Can you work these out from the model? Positions are in its coordinate system, mm. Round coordinates to 2 decimals unless told otherwise and drop trailing zeros. Loops run counter-clockwise (first coordinate to the right, second up) from the corner with the lowest first, then second, coordinate; pieces in that order, holes last. Notation, with made-up numbers: (62, 40.5) -> (98, 40.5) arc R9 cw to (98, 57.5) -> close; hole circle Ø4 at (27.5, 11). An arc over 180 degrees is marked (long way). Answer as a JSON object with one key per item and string values.
```python
from build123d import *

# Parameters (mm, degrees)
SKETCH_1_W          = 130
SKETCH_1_H          = 130
EXTRUDE_1_DEPTH     = 3
SKETCH_5_R          = 2
CUT_EXTRUDE_4_DEPTH = 3
SKETCH_6_R          = 1.5
SKETCH_6_R_2        = 1.464964174
CUT_EXTRUDE_5_DEPTH = 10


with BuildPart() as part:
    # 草图1 → 凸台-拉伸1 (new body)
    with BuildSketch(Plane.XY):
        Rectangle(SKETCH_1_W, SKETCH_1_H)
    extrude(amount=EXTRUDE_1_DEPTH)

    # 草图5 → 切除-拉伸4 (cut)
    with BuildSketch(Plane.XY.offset(3)):
        with Locations((25, -25)):
            Circle(SKETCH_5_R)
        with Locations((-25, 25)):
            Circle(SKETCH_5_R)
    extrude(amount=-CUT_EXTRUDE_4_DEPTH, mode=Mode.SUBTRACT)

    # 草图6 → 切除-拉伸5 (cut)
    with BuildSketch(Plane.XY.offset(3)):
        with Locations((-54.393398282, 54.393398282)):
            Circle(SKETCH_6_R)
        with Locations((-43.786796564, 43.786796564)):
            Circle(SKETCH_6_R)
        with Locations((-10.232887384, 47)):
            Circle(SKETCH_6_R)
        with Locations((9.767112616, 47)):
            Circle(SKETCH_6_R)
        with Locations((43.786796564, 43.786796564)):
            Circle(SKETCH_6_R)
        with Locations((54.393398282, 54.393398282)):
            Circle(SKETCH_6_R)
        with Locations((-47, 10)):
            Circle(SKETCH_6_R)
        with Locations((-47, -10)):
            Circle(SKETCH_6_R)
        with Locations((47, -10)):
            Circle(SKETCH_6_R)
        with Locations((47, 10)):
            Circle(SKETCH_6_R)
        with Locations((-54.393398282, -54.393398282)):
            Circle(SKETCH_6_R)
        with Locations((-43.786796564, -43.786796564)):
            Circle(SKETCH_6_R)
        with Locations((-10, -47)):
            Circle(SKETCH_6_R_2)
        with Locations((10, -47)):
            Circle(SKETCH_6_R)
        with Locations((43.786796564, -43.786796564)):
            Circle(SKETCH_6_R)
        with Locations((54.393398282, -54.393398282)):
            Circle(SKETCH_6_R)
    extrude(amount=-CUT_EXTRUDE_5_DEPTH, mode=Mode.SUBTRACT)


solid = part.part
```
Q1. We'd pull the mould along Y, two halves only. Please class faces 1 (the flat face through (-1, 65, 1)), 2 (the cylindrical face through (-10.191, -45.548, 1.521)), 3 (the cylindrical face through (45.5, 10.07, 1.52)), 4 (the flat face through (-1, 1, 0)): pulls with the +Y half, pulls with the -Y half, needs draft (parallel to the pull), parting line crosses it, or undercut.
Determined:
{"face 1": "pulls with the +Y half", "face 2": "undercut", "face 3": "undercut", "face 4": "needs draft"}
Q2. I want a section at B-B, the plane x = 25. Write out the boundary of the cut face in (y, z), then the cut area to 3 significant figures.
Determined:
{"outline": "(-65, 0) -> (-27, 0) -> (-27, 3) -> (-65, 3) -> close; (-23, 0) -> (65, 0) -> (65, 3) -> (-23, 3) -> close", "area": "378 mm²"}
Q3. If I drill on L1, parallel to Y at x = -47, z = 1.75; L2, parallel to X at y = 54.5, z = 1.35; L3, parallel to Y at x = -25, z = 1.6, over which ranges is the centre line in solid material (lowest first)? Write a range as [from, to].
Determined:
{"L1": "[-65, -11.5], [-8.5, 8.5], [11.5, 65]", "L2": "[-65, -55.89], [-52.9, 52.9], [55.89, 65]", "L3": "[-65, 23], [27, 65]"}
Q4. I want a section at C-C, the plane y = 10. Write out the boundary of the cut face in (x, z).
Determined:
{"outline": "(-65, 0) -> (-48.5, 0) -> (-48.5, 3) -> (-65, 3) -> close; (-45.5, 0) -> (45.5, 0) -> (45.5, 3) -> (-45.5, 3) -> close; (48.5, 0) -> (65, 0) -> (65, 3) -> (48.5, 3) -> close"}
Q5. I'm going to push a flat-ended pin straight in: pin 1 (1.5 mm diameter, centred on x = -17.5, y = 10, fed in from -Z). Where does the tip first touch, or does it pass through?
Determined:
{"pin 1": "z = 0"}
Q6. I want a section at A-A, the plane y = -25. Write out the boundary of the cut face in (x, z).
Determined:
{"outline": "(-65, 0) -> (23, 0) -> (23, 3) -> (-65, 3) -> close; (27, 0) -> (65, 0) -> (65, 3) -> (27, 3) -> close"}
